Autodesk Inventor part; units mm, degrees
ref_plane "YZ Plane" through (0, 0, 0) normal (1, 0, 0) x (0, 1, 0)
ref_plane "XZ Plane" through (0, 0, 0) normal (0, 1, 0) x (-1, 0, 0)
ref_plane "XY Plane" through (0, 0, 0) normal (0, 0, 1) x (1, 0, 0)
sketch "Szkic1" plane through (0, 0, 0) normal (0, 0, 1) x (1, 0, 0)
  circle A0 centre (0, 0) radius 32.5
  dimension "d0" = 65
extrude "Wyciągnięcie proste1" add sketch "Szkic1" along normal blind 164
sketch "Szkic2" plane through (0, 0, 0) normal (0, 0, -1) x (-1, 0, 0)
  circle A0 centre (0, 0) radius 32.5
  circle A1 centre (0, 0) radius 33
  dimension "d3" = 66
extrude "Wyciągnięcie proste2" add sketch "Szkic2" along normal blind 25 contours A0 | A1
sketch "Szkic3" plane through (0, 0, 164) normal (0, 0, 1) x (1, 0, 0)
  circle A0 centre (0, 0) radius 33
  dimension "d6" = 66
extrude "Wyciągnięcie proste3" add sketch "Szkic3" along normal blind 8
sketch "Szkic4" plane through (0, 0, 172) normal (0, 0, 1) x (1, 0, 0)
  circle A0 centre (0, 0) radius 22
  dimension "d9" = 44
extrude "Wyciągnięcie proste4" add sketch "Szkic4" along normal blind 22
sketch "Szkic5" plane through (0, 0, 194) normal (0, 0, 1) x (1, 0, 0)
  circle A0 centre (0, 0) radius 9.5
  dimension "d12" = 19
extrude "Wyciągnięcie proste5" add sketch "Szkic5" along normal blind 36
sketch "Szkic6" plane through (0, 0, 230) normal (0, 0, 1) x (1, 0, 0)
  circle A0 centre (0, 0) radius 4
  dimension "d15" = 8
extrude "Wyciągnięcie proste6" cut sketch "Szkic6" against normal blind 30
properties part number "Wrzeciono Elektrowrzeciono CNC 0.8kw"
The model under review builds one solid part; all positions refer to its coordinate system, in mm. A direction names the side the tool comes from. Give positions to 0.01 mm unless a question says otherwise; leave off trailing zeros. Loops run counter-clockwise (first coordinate to the right, second up) from the corner with the lowest first, then second, coordinate; pieces in that order, holes last. Notation, with made-up numbers: (48.25, 89.25) -> (69.25, 89.25) arc R7 ccw to (69.25, 96.25) -> close; hole circle Ø3 at (-16.75, 25.5). An arc over 180 degrees is marked (long way). Put each result on its own line as item: value. Start each with the question number.
1. Mouldability with a two-part tool opening along Z and no side actions: class faces 4 (the face through (0, 0, -25)), 5 (the face through (24.29, -21.85, 164)), 6 (the face through (-24.29, -21.85, 0)), 7 (the face through (4.38, 8.43, 211.75)) as released by +Z, released by -Z, zero draft, split by the parting line, or undercut.
2. Wall thickness on probe 1 along Y at (x, z) = (0, 216); probe 2 along Z at (x, y) = (-3, 21.5); probe 3 along Z at (x, y) = (-20, 20.5): over which ranges is each line inside the solid? List them lowest first.
3. We need section D-D on y = -16.5. State the section outline as (x, z) points.
4. For faces 1 (the face through (-0.867, -3.905, 215.21)), 2 (the face through (31, -9.76, 80.85)), 3 (the face through (30.5, 12.6, 167.9)), list the 3-axis set-ups (+Z, -Z, +X, -X, +Y, -Y) from which the entire face can be reached by the end or side of a thin tool; tool diameter is ignored.
5. Clearance check with flat-ended pins moving along their axes: P1, Ø5, axis at x = 26, z = 90.5, coming from the -Y side; P2, Ø8, axis at y = 6.5, z = 40.5, coming from the -X side; P3, Ø4, axis at x = -23, z = 88, coming from the +Y side. State where each tip first meets the part, or that it passes through.
6. We need section A-A on x = 0. State the section outline as (y, z) points, then the cut area to 4 significant figures.
7. We need section C-C on z = 41.5. State the section outline as (x, y) points.
Determined:
1. face 4: released by -Z
1. face 5: undercut
1. face 6: undercut
1. face 7: zero draft
2. probe 1: -9.5 to -4, 4 to 9.5
2. probe 2: -25 to 194
2. probe 3: -25 to 172
3. outline: (-28.58, -25) -> (28.58, -25) -> (28.58, 0) -> (28, 0) -> (28, 164) -> (28.58, 164) -> (28.58, 172) -> (14.55, 172) -> (14.55, 194) -> (-14.55, 194) -> (-14.55, 172) -> (-28.58, 172) -> (-28.58, 164) -> (-28, 164) -> (-28, 0) -> (-28.58, 0) -> close
4. face 1: +Z
4. face 2: none
4. face 3: +Z, -Z
5. P1: y = -22.45
5. P2: x = -32.4
5. P3: y = 24.8
6. outline: (-33, -25) -> (33, -25) -> (33, 0) -> (32.5, 0) -> (32.5, 164) -> (33, 164) -> (33, 172) -> (22, 172) -> (22, 194) -> (9.5, 194) -> (9.5, 230) -> (4, 230) -> (4, 200) -> (-4, 200) -> (-4, 230) -> (-9.5, 230) -> (-9.5, 194) -> (-22, 194) -> (-22, 172) -> (-33, 172) -> (-33, 164) -> (-32.5, 164) -> (-32.5, 0) -> (-33, 0) -> close
6. area: 14,250 mm^2
7. outline: circle Ø65 at (0, 0)
